Check sheet for the drawn part. Datum: minimum x, y, z corner. Units: mm. Round coordinates to 2 decimals unless told otherwise and drop trailing zeros. Write each loop counter-clockwise with the first axis right and the second up, starting at its lowest first coordinate (ties: lowest second). Pieces come first, ordered by that corner, then holes.
Item 1: Cross-section at A-A on y = 719.5. Enter the section's corners in (x, z), plus the area to 3 significant figures.
Item 2: Release check for a two-part mould opening along X. For the marked faces 1 and 2 record: +X half, -X half, draft (parallel to the pull), parting line (faces both ways), or undercut.
Item 3: Cross-section at B-B on z = 1072.5. Enter the section's corners in (x, y).
Item 4: Go/stop test with flat-tipped pins: pin 1 Ø12.5 at (x, y) = (10.5, 185.5) entering from -Z; pin 2 Ø7.5 at (x, z) = (19, 1690.5) entering from -Y; pin 3 Ø3 at (x, y) = (22.5, 249.5) entering from +Z. Record where each tip stops, or that it passes through.
Item 5: Material ranges on line 1 (Z direction, x = 19.5, y = 809.5); line 2 (Y direction, x = 4.5, z = 855), recorded low to high.
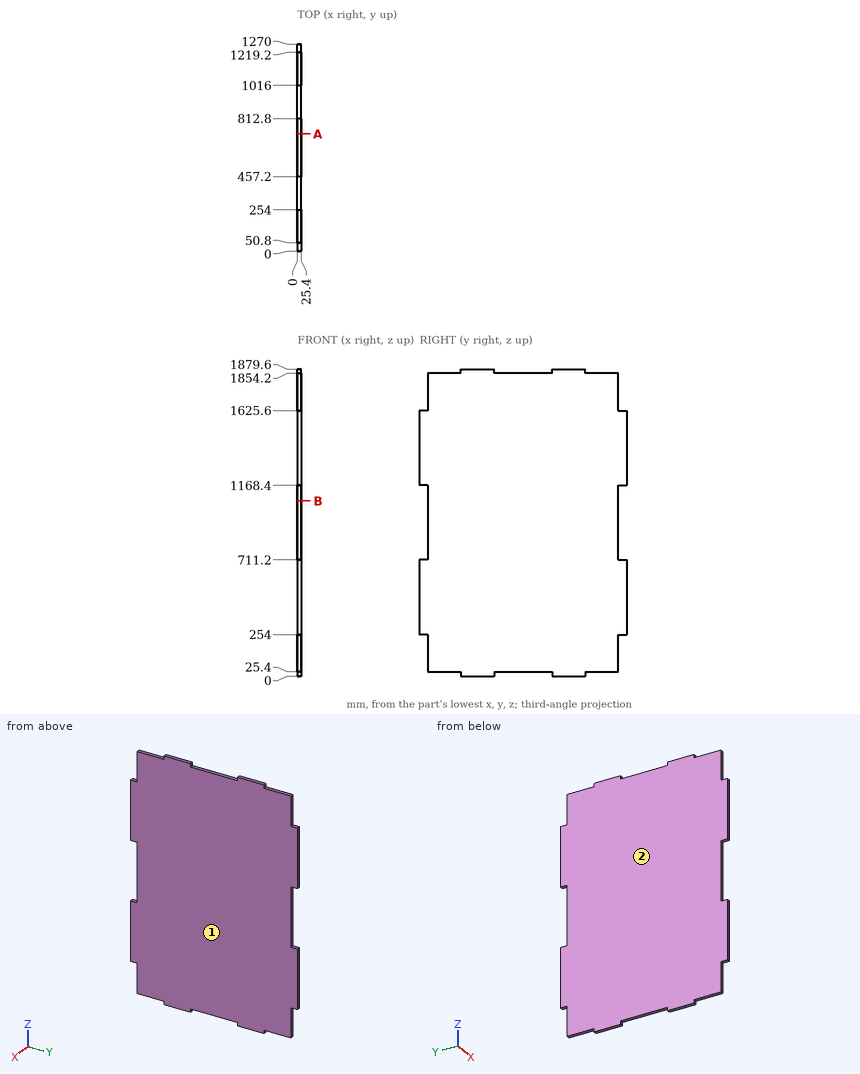
Response values:
1. outline: (0, 25.4) - (25.4, 25.4) - (25.4, 1854.2) - (0, 1854.2) - close
1. area: 46,500 mm2
2. face 1: +X half
2. face 2: -X half
3. outline: (0, 50.8) - (25.4, 50.8) - (25.4, 1219.2) - (0, 1219.2) - close
4. pin 1: stops at z = 25.4
4. pin 2: stops at y = 50.8
4. pin 3: stops at z = 1854.2
5. line 1: z = 25.4 to 1854.2
5. line 2: y = 50.8 to 1219.2
